```python
from build123d import *

# Parameters (mm, degrees)
EXTRUDE_1_DEPTH = 0.3
CHAMFER_1_SIZE  = 0.05


with BuildPart() as part:
    # 草图1 → 凸台-拉伸1 (new body)
    with BuildSketch(Plane.XY):
        with BuildLine():
            ThreePointArc((-1.295808382, 0.104310288), (-1.288091369, -0.175558041), (-1.220629908, -0.44728361))
            ThreePointArc((-1.220629908, -0.44728361), (-1.21876562, -1.508256965), (-1.9, -2.321637353))
            ThreePointArc((-1.9, -2.321637353), (0, 3), (1.9, -2.321637353))
            ThreePointArc((1.9, -2.321637353), (1.21876562, -1.508256965), (1.220629908, -0.44728361))
            ThreePointArc((1.220629908, -0.44728361), (1.288091369, -0.175558041), (1.295808382, 0.104310288))
            ThreePointArc((1.295808382, 0.104310288), (1.625, 1.077903057), (0.600024951, 1.153243278))
            ThreePointArc((0.600024951, 1.153243278), (0, 1.3), (-0.600024951, 1.153243278))
            ThreePointArc((-0.600024951, 1.153243278), (-1.625, 1.077903057), (-1.295808382, 0.104310288))
        make_face()
    extrude(amount=EXTRUDE_1_DEPTH)

    # 倒角1
    chamfer_1_edges = [part.edges().sort_by_distance(p)[0] for p in [
        (0, 3, 0.3),
        (0, 3, 0),
    ]]
    chamfer(chamfer_1_edges, length=CHAMFER_1_SIZE)


solid = part.part
```
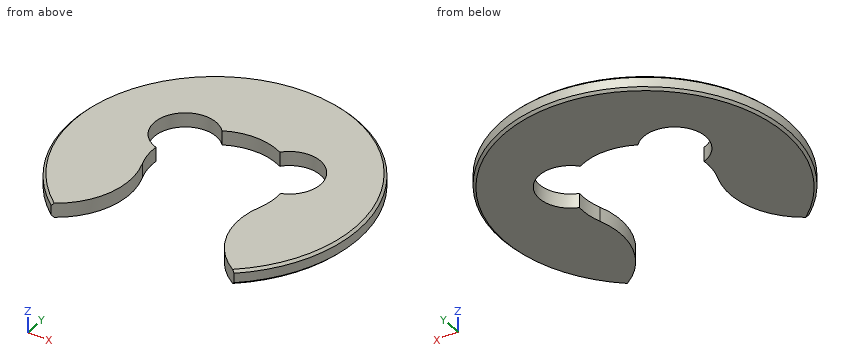
Geometry check sheet. Reference: the model listing, model coordinates, mm. Round coordinates to 2 decimals unless told otherwise and drop trailing zeros. Loops run counter-clockwise (first coordinate to the right, second up) from the corner with the lowest first, then second, coordinate; pieces in that order, holes last. Notation, with made-up numbers: (71, 40) - (85, 40) arc R22 ccw to (85, 51) - close; hole circle Ø5 at (58.25, 88.25). An arc over 180 degrees is marked (long way). Write item = value, one per line. Start each with the question number.
1. Depth check by flat-ended pin: pin 1 (2 mm diameter, centred on x = 0, y = 0.5, fed in from -Z). Enter the tip coordinate at first touch or a pass-through.
2. Section check A-A on y = 0. Enter the section's corners in (x, z), then the cut area to 4 significant figures.
3. Section check B-B on x = 0. Enter the section's corners in (y, z).
4. Thickness scan on line 1 (X direction, y = -0.05, z = 0.2); line 2 (X direction, y = -1.8, z = 0.2); line 3 (Y direction, x = 1.5, z = 0.15). Record the ranges inside material, lowest first.
5. Section check C-C on z = 0.2. Enter the section's corners in (x, y).
Working result:
q1.pin_1 = 0
q2.outline = (-3, 0.05) - (-2.95, 0) - (-1.3, 0) - (-1.3, 0.3) - (-2.95, 0.3) - (-3, 0.25) - close; (1.3, 0) - (2.95, 0) - (3, 0.05) - (3, 0.25) - (2.95, 0.3) - (1.3, 0.3) - close
q2.area = 1.015 mm^2
q3.outline = (1.3, 0) - (2.95, 0) - (3, 0.05) - (3, 0.25) - (2.95, 0.3) - (1.3, 0.3) - close
q4.line_1 = -3 to -1.3, 1.3 to 3
q4.line_2 = -2.4 to -1.36, 1.36 to 2.4
q4.line_3 = -1.99 to 0.22, 1.22 to 2.6
q5.outline = (-1.9, -2.32) arc R1.55 ccw to (-1.22, -0.45) arc R1.3 cw to (-1.3, 0.1) arc R0.65 cw (long way) to (-0.6, 1.15) arc R1.3 cw to (0.6, 1.15) arc R0.65 cw (long way) to (1.3, 0.1) arc R1.3 cw to (1.22, -0.45) arc R1.55 ccw to (1.9, -2.32) arc R3 ccw (long way) to start
